from build123d import *

# Parameters (mm, degrees)
BOX001_W      = 20
BOX001_H      = 10
BOX001_DEPTH  = 10
TUBE001_R     = 7.2
TUBE001_R_2   = 6.2
TUBE001_DEPTH = 10
BOX_W         = 10
BOX_H         = 10
BOX_DEPTH     = 10
TUBE_R        = 3.8
TUBE_R_2      = 2.9
TUBE_DEPTH    = 10


with BuildPart() as cube001:
    # Box001 → Box001 (new body)
    with BuildSketch(Plane(origin=(-10, -15, 0), x_dir=(1, 0, 0), z_dir=(0, 0, 1))):
        with Locations((10, 5)):
            Rectangle(BOX001_W, BOX001_H)
    extrude(amount=BOX001_DEPTH)


with BuildPart() as cut001:
    # Tube001 → Tube001 (new body)
    with BuildSketch(Plane.XY):
        Circle(TUBE001_R)
        Circle(TUBE001_R_2, mode=Mode.SUBTRACT)
    extrude(amount=TUBE001_DEPTH)

    # Cut001: cut Cube001
    add(cube001.part, mode=Mode.SUBTRACT)


with BuildPart() as cube:
    # Box → Box (new body)
    with BuildSketch(Plane(origin=(-5, 12.6, 0), x_dir=(1, 0, 0), z_dir=(0, 0, 1))):
        with Locations((5, 5)):
            Rectangle(BOX_W, BOX_H)
    extrude(amount=BOX_DEPTH)


with BuildPart() as fusion:
    # Tube → Tube (new body)
    with BuildSketch(Plane(origin=(0, 10.1, 0), x_dir=(1, 0, 0), z_dir=(0, 0, 1))):
        Circle(TUBE_R)
        Circle(TUBE_R_2, mode=Mode.SUBTRACT)
    extrude(amount=TUBE_DEPTH)

    # Cut: cut Cube
    add(cube.part, mode=Mode.SUBTRACT)

    # Fusion: union Cut001
    add(cut001.part)


solid = fusion.part
Could you check a few things on this model? Use its own coordinates, in mm. Round coordinates to 2 decimals unless told otherwise and drop trailing zeros. Write each loop counter-clockwise with the first axis right and the second up, starting at its lowest first coordinate (ties: lowest second). Pieces come first, ordered by that corner, then holes. Notation, with made-up numbers: (23.25, -7.5) - (41.25, -7.5) arc R16 cw to (41.25, 11.5) - close; hole circle Ø2 at (-13.75, 75.5). An arc over 180 degrees is marked (long way). Put each result on its own line as item: value. Start each with the question number.
(1) I want a section at C-C, the plane z = 3.5. Please give me the cut outline in (x, y).
(2) Will this pin go through, and if not, where does the flat tip stop? pin 1 (3.5 mm diameter, centred on x = 0, y = 10.1, fed in from -Z).
(3) I want a section at D-D, the plane x = 0. Please give me the cut outline in (y, z), plus the area to 4 significant figures.
(4) Thinking about a two-plate mould opening in Y: for faces 1 (the flat face through (0, 6.4, 10)), 2 (the cylindrical face through (-0.1, 7.2, 4.9)), 3 (the cylindrical face through (-3.77, 9.61, 4.93)), 4 (the flat face through (2, 12.6, 5)), which applies, released by +Y, released by -Y, zero draft, split by the parting line, or undercut?
(5) I want a section at A-A, the plane y = 5. Please give me the cut outline in (x, z), plus the area to 3 significant figures.
(6) I need wall thicknesses on probe 1 along X at (y, z) = (10.25, 6.25); probe 2 along X at (y, z) = (0, 3); probe 3 along Y at (x, z) = (2.25, 4.75). Which ranges of each line are inside material? Lowest first, please.
(7) I want a section at B-B, the plane x = 4.75. Please give me the cut outline in (y, z), plus the area to 3 significant figures.
Here are the results:
1. outline: (-5.18, -5) - (-3.67, -5) arc R6.2 cw (long way) to (3.67, -5) - (5.18, -5) arc R7.2 ccw to (2.05, 6.9) arc R3.8 ccw to (2.86, 12.6) - (1.47, 12.6) arc R2.9 cw (long way) to (-1.47, 12.6) - (-2.86, 12.6) arc R3.8 ccw to (-2.05, 6.9) arc R7.2 ccw to start
2. pin 1: passes through
3. outline: (6.2, 0) - (7.2, 0) - (7.2, 10) - (6.2, 10) - close
3. area: 10.00 mm^2
4. face 1: zero draft
4. face 2: undercut
4. face 3: undercut
4. face 4: released by +Y
5. outline: (-5.18, 0) - (-3.67, 0) - (-3.67, 10) - (-5.18, 10) - close; (3.67, 0) - (5.18, 0) - (5.18, 10) - (3.67, 10) - close
5. area: 30.3 mm^2
6. probe 1: x = -3.8 to -2.9, 2.9 to 3.8
6. probe 2: x = -7.2 to -6.2, 6.2 to 7.2
6. probe 3: y = 5.78 to 6.84, 7.04 to 8.27, 11.93 to 12.6
7. outline: (-5, 0) - (-3.98, 0) - (-3.98, 10) - (-5, 10) - close; (3.98, 0) - (5.41, 0) - (5.41, 10) - (3.98, 10) - close
7. area: 24.4 mm^2
